from build123d import *

# Parameters (mm, degrees)
BOX_EXTRUDE_DEPTH                = 12.5
SHELL1_T                         = -3
CUT_SWEEP_START                  = -12.5
CUT_SWEEP_DEPTH                  = 4.5
SKETCH2_W                        = 10
SKETCH2_H                        = 10
SQUARES_EXTRUDE_DEPTH            = 9.5
SKETCH11_W                       = 10
SKETCH11_H                       = 31
SKETCH11_W_2                     = 45
SKETCH11_H_2                     = 10
CUT_EXTRUDE2_DEPTH               = 214.65503369
SQUARES_M3_CLEARANCE_HOLES_D     = 2.5
SQUARES_M3_CLEARANCE_HOLES_DEPTH = 2
SQUARES_M3_CLEARANCE_HOLES_TIP   = 0.751075774
F_8_0MM_DOWEL_HOLE1_D            = 8
F_8_0MM_DOWEL_HOLE1_DEPTH        = 7.5
F_8_0MM_DOWEL_HOLE1_TIP          = 2.403442476
F_5_0MM_DOWEL_HOLE1_D            = 5
F_5_0MM_DOWEL_HOLE1_DEPTH        = 7.5
F_5_0MM_DOWEL_HOLE1_TIP          = 1.502151548
M3_CLEARANCE_HOLE3_D             = 3.4
M3_CLEARANCE_HOLE3_DEPTH         = 7.5
M3_CLEARANCE_HOLE3_TIP           = 1.021463052
M3_5X0_6_TAPPED_HOLE1_D          = 2.9
M3_5X0_6_TAPPED_HOLE2_D          = 2.9
M3_5X0_6_TAPPED_HOLE2_DEPTH      = 8.8
M3_5X0_6_TAPPED_HOLE2_TIP        = 0.871247898
SKETCH25_W                       = 3
SKETCH25_H                       = 31
BOSS_EXTRUDE1_DEPTH              = 38.75
F_2_5MM_DOWEL_HOLE1_D            = 2.5
F_2_5MM_DOWEL_HOLE1_DEPTH        = 10
F_2_5MM_DOWEL_HOLE1_TIP          = 0.751075774


# Read off the part's stored shape, not the designer's step: Cut-Sweep
with BuildPart() as part:
    # Sketch1 → Box-Extrude (new body)
    with BuildSketch(Plane.XY):
        with BuildLine():
            Line((-64.633571826, -98.481365252), (179.366428174, -98.481365252))
            ThreePointArc((179.366428174, -98.481365252), (186.437495986, -95.552433064), (189.366428174, -88.481365252))
            Line((189.366428174, -88.481365252), (189.366428174, -8.481365252))
            ThreePointArc((189.366428174, -8.481365252), (186.437495986, -1.41029744), (179.366428174, 1.518634748))
            Line((179.366428174, 1.518634748), (-64.633571826, 1.518634748))
            ThreePointArc((-64.633571826, 1.518634748), (-71.704639638, -1.41029744), (-74.633571826, -8.481365252))
            Line((-74.633571826, -8.481365252), (-74.633571826, -88.481365252))
            ThreePointArc((-74.633571826, -88.481365252), (-71.704639638, -95.552433064), (-64.633571826, -98.481365252))
        make_face()
    extrude(amount=-BOX_EXTRUDE_DEPTH)

    # Shell1
    shell1_openings = [part.faces().sort_by_distance(p)[0] for p in [
        (57.366428174, -48.481365252, -12.5),
    ]]
    offset(amount=SHELL1_T, openings=shell1_openings, kind=Kind.INTERSECTION)

    # Cut-Sweep outline → Cut-Sweep (cut)
    with BuildSketch(Plane.XY.offset(CUT_SWEEP_START)):
        with BuildLine():
            Line((189.366428174, -88.481365252), (189.366428174, -8.481365252))
            ThreePointArc((189.366428174, -8.481365252), (186.437495986, -1.41029744), (179.366428174, 1.518634748))
            Line((179.366428174, 1.518634748), (-64.633571826, 1.518634748))
            ThreePointArc((-64.633571826, 1.518634748), (-71.704639638, -1.41029744), (-74.633571826, -8.481365252))
            Line((-74.633571826, -8.481365252), (-74.633571826, -88.481365252))
            ThreePointArc((-74.633571826, -88.481365252), (-71.704639638, -95.552433064), (-64.633571826, -98.481365252))
            Line((-64.633571826, -98.481365252), (179.366428174, -98.481365252))
            ThreePointArc((179.366428174, -98.481365252), (186.437495986, -95.552433064), (189.366428174, -88.481365252))
        make_face()
        with BuildLine():
            Line((179.366428174, -96.981365252), (-64.633571826, -96.981365252))
            ThreePointArc((-64.633571826, -96.981365252), (-70.643979466, -94.491772892), (-73.133571826, -88.481365252))
            Line((-73.133571826, -88.481365252), (-73.133571826, -8.481365252))
            ThreePointArc((-73.133571826, -8.481365252), (-70.643979466, -2.470957612), (-64.633571826, 0.018634748))
            Line((-64.633571826, 0.018634748), (179.366428174, 0.018634748))
            ThreePointArc((179.366428174, 0.018634748), (185.376835814, -2.470957612), (187.866428174, -8.481365252))
            Line((187.866428174, -8.481365252), (187.866428174, -88.481365252))
            ThreePointArc((187.866428174, -88.481365252), (185.376835814, -94.491772892), (179.366428174, -96.981365252))
        make_face(mode=Mode.SUBTRACT)
    extrude(amount=CUT_SWEEP_DEPTH, mode=Mode.SUBTRACT)

    # Sketch2 → Squares-Extrude (add)
    with BuildSketch(Plane.XY.offset(-3)):
        with Locations((41.816428174, -6.481365252)):
            Rectangle(SKETCH2_W, SKETCH2_H)
        with Locations((181.366428174, -65.481365252)):
            Rectangle(SKETCH2_W, SKETCH2_H)
        with Locations((41.366428174, -90.481365252)):
            Rectangle(SKETCH2_W, SKETCH2_H)
        with Locations((181.366428174, -31.481365252)):
            Rectangle(SKETCH2_W, SKETCH2_H)
    extrude(amount=-SQUARES_EXTRUDE_DEPTH)

    # Sketch11 → Cut-Extrude2 (cut, through all)
    with BuildSketch(Plane(origin=(0, 0, -3), x_dir=(-1, 0, 0), z_dir=(0, 0, -1))):
        with BuildLine():
            Line((-166.366428174, -66.481365252), (-110.366428174, -66.481365252))
            ThreePointArc((-110.366428174, -66.481365252), (-108.952214612, -65.895578814), (-108.366428174, -64.481365252))
            Line((-108.366428174, -64.481365252), (-108.366428174, -28.481365252))
            ThreePointArc((-108.366428174, -28.481365252), (-108.952214612, -27.067151689), (-110.366428174, -26.481365252))
            Line((-110.366428174, -26.481365252), (-166.366428174, -26.481365252))
            ThreePointArc((-166.366428174, -26.481365252), (-167.780641736, -27.067151689), (-168.366428174, -28.481365252))
            Line((-168.366428174, -28.481365252), (-168.366428174, -64.481365252))
            ThreePointArc((-168.366428174, -64.481365252), (-167.780641736, -65.895578814), (-166.366428174, -66.481365252))
        make_face()
        with Locations((62.633571826, -44.311365252)):
            Rectangle(SKETCH11_W, SKETCH11_H)
        with Locations((-152.769428174, 113.518634748)):
            Rectangle(SKETCH11_W_2, SKETCH11_H_2)
    extrude(amount=-CUT_EXTRUDE2_DEPTH, mode=Mode.SUBTRACT)

    # Squares M3 Clearance Holes
    with Locations(Plane(origin=(0, 0, -12.5), x_dir=(1, 0, 0), z_dir=(0, 0, -1))):
        with Locations((41.816428174, 6.481365252), (181.366428174, 31.481365252), (181.366428174, 65.481365252), (41.366428174, 90.481365252)):
            Hole(SQUARES_M3_CLEARANCE_HOLES_D / 2, depth=SQUARES_M3_CLEARANCE_HOLES_DEPTH)
            with Locations((0, 0, -(SQUARES_M3_CLEARANCE_HOLES_DEPTH + SQUARES_M3_CLEARANCE_HOLES_TIP / 2))):  # 118° drill point
                Cone(0, SQUARES_M3_CLEARANCE_HOLES_D / 2, SQUARES_M3_CLEARANCE_HOLES_TIP, mode=Mode.SUBTRACT)

    # Ø8.0mm Dowel Hole1
    with Locations(Plane(origin=(169.366428174, -85.481365252, -3), x_dir=(-1, 0, 0), z_dir=(0, 0, -1))):
        with Locations((0, 0), (31, 0), (62, 0), (71, 67), (-9, 67)):
            Hole(F_8_0MM_DOWEL_HOLE1_D / 2, depth=F_8_0MM_DOWEL_HOLE1_DEPTH)
            with Locations((0, 0, -(F_8_0MM_DOWEL_HOLE1_DEPTH + F_8_0MM_DOWEL_HOLE1_TIP / 2))):  # 118° drill point
                Cone(0, F_8_0MM_DOWEL_HOLE1_D / 2, F_8_0MM_DOWEL_HOLE1_TIP, mode=Mode.SUBTRACT)

    # Ø5.0mm Dowel Hole1
    with Locations(Plane(origin=(0, 0, -3), x_dir=(-1, 0, 0), z_dir=(0, 0, -1))):
        with Locations((-138.366428174, -22.481365252)):
            Hole(F_5_0MM_DOWEL_HOLE1_D / 2, depth=F_5_0MM_DOWEL_HOLE1_DEPTH)
            with Locations((0, 0, -(F_5_0MM_DOWEL_HOLE1_DEPTH + F_5_0MM_DOWEL_HOLE1_TIP / 2))):  # 118° drill point
                Cone(0, F_5_0MM_DOWEL_HOLE1_D / 2, F_5_0MM_DOWEL_HOLE1_TIP, mode=Mode.SUBTRACT)

    # M3 Clearance Hole3
    with Locations(Plane(origin=(0, 0, -3), x_dir=(-1, 0, 0), z_dir=(0, 0, -1))):
        with Locations((-163.366428174, -15.481365252), (-113.366428174, -15.481365252), (-163.366428174, -92.481365252), (-113.366428174, -92.481365252)):
            Hole(M3_CLEARANCE_HOLE3_D / 2, depth=M3_CLEARANCE_HOLE3_DEPTH)
            with Locations((0, 0, -(M3_CLEARANCE_HOLE3_DEPTH + M3_CLEARANCE_HOLE3_TIP / 2))):  # 118° drill point
                Cone(0, M3_CLEARANCE_HOLE3_D / 2, M3_CLEARANCE_HOLE3_TIP, mode=Mode.SUBTRACT)

    # M3.5x0.6 Tapped Hole1 (through all)
    with Locations(Plane(origin=(0, 0, -3), x_dir=(-1, 0, 0), z_dir=(0, 0, -1))):
        with Locations((-172.205915164, -24.061365252), (-172.205915164, -66.561365252), (-89.226428174, -25.561365252), (-89.226428174, -65.061365252), (-171.219428174, -11.481365252), (-131.719428174, -11.481365252)):
            Hole(M3_5X0_6_TAPPED_HOLE1_D / 2)

    # M3.5x0.6 Tapped Hole2
    with Locations(Plane.XY):
        with Locations((-66.633571826, -8.481365252), (-66.633571826, -88.481365252)):
            Hole(M3_5X0_6_TAPPED_HOLE2_D / 2, depth=M3_5X0_6_TAPPED_HOLE2_DEPTH)
            with Locations((0, 0, -(M3_5X0_6_TAPPED_HOLE2_DEPTH + M3_5X0_6_TAPPED_HOLE2_TIP / 2))):  # 118° drill point
                Cone(0, M3_5X0_6_TAPPED_HOLE2_D / 2, M3_5X0_6_TAPPED_HOLE2_TIP, mode=Mode.SUBTRACT)

    # Sketch25 → Boss-Extrude1 (add)
    with BuildSketch(Plane(origin=(0, 0, -3), x_dir=(-1, 0, 0), z_dir=(0, 0, -1))):
        with Locations((56.133571826, -44.311365252)):
            Rectangle(SKETCH25_W, SKETCH25_H)
    extrude(amount=BOSS_EXTRUDE1_DEPTH)

    # Ø2.5mm Dowel Hole1
    with Locations(Plane(origin=(-54.633571826, 0, 0), x_dir=(0, 0, -1), z_dir=(1, 0, 0))):
        with Locations((37.25, -32.811365252), (37.25, -55.811365252), (14.25, -32.811365252), (14.25, -55.811365252)):
            Hole(F_2_5MM_DOWEL_HOLE1_D / 2, depth=F_2_5MM_DOWEL_HOLE1_DEPTH)
            with Locations((0, 0, -(F_2_5MM_DOWEL_HOLE1_DEPTH + F_2_5MM_DOWEL_HOLE1_TIP / 2))):  # 118° drill point
                Cone(0, F_2_5MM_DOWEL_HOLE1_D / 2, F_2_5MM_DOWEL_HOLE1_TIP, mode=Mode.SUBTRACT)


solid = part.part
For this review, take the finished solid that the model builds, in its own axes (mm). A direction names the side the tool comes from. Give positions to 0.01 mm unless a question says otherwise; leave off trailing zeros. Loops run counter-clockwise (first coordinate to the right, second up) from the corner with the lowest first, then second, coordinate; pieces in that order, holes last. Notation, with made-up numbers: M -32,30 L -13,30 A25 cw -13,52 Z; hole C 87,41.25 d2. An arc over 180 degrees is marked long. Answer as a JSON object with one key per item and string values. Group by question number.
Q1. For probe 1 along X at (y, z) = (-47, -4.5); probe 2 along X at (y, z) = (-40.5, -10); probe 3 along Y at (x, z) = (-55, -14), list the stretches that pass through material, from the lowest coordinate up. Write a range as [from, to].
Q2. Add section C-C on z = -29. Give the boundary of the cut face in (x, y), and give its area (3 significant figures).
Q3. Tool access review of faces 1 (the flat face through (181, -36.481, -8)), 2 (the flat face through (-57.634, -45, -21)), 3 (the cylindrical face through (-70.71, -2.54, -10.28)), 4 (the flat face through (56, 0.019, -10)): name each direction out of +Z, -Z, +X, -X, +Y, -Y from which nothing blocks a thin tool from reaching the whole face with its end or side.
Q4. Insertion check: P1, Ø5, axis at x = 182.5, z = -6, coming from the +Y side; P2, Ø8, axis at x = 29.5, z = -16, coming from the +Y side; P3, Ø3, axis at y = -6, z = -8.5, coming from the +X side; P4, Ø6, axis at y = -25, z = -21.5, coming from the +X side. Each pin has a flat end and moves straight along its axis. Give the tip position at first contact, or say it passes through.
Q5. Add section B-B on x = 70.5. Give the boundary of the cut face in (y, z).
Q6. Mouldability with a two-part tool opening along X and no side actions: class faces 5 (the flat face through (59, 1.519, -4)), 6 (the flat face through (176.366, -32, -8)), 7 (the flat face through (187.866, -48, -10)), 8 (the flat face through (-73.134, -49, -10)) as +X half, -X half, draft (parallel to the pull), parting line (faces both ways), or undercut.
Q7. Add section A-A on y = -49.5. Give the boundary of the cut face in (x, z).
Checked values:
{
 "1": {"probe 1": "[-74.63, -71.63], [-57.63, -54.63], [186.37, 189.37]", "probe 2": "[-73.13, -71.63], [-57.63, -54.63], [186.37, 187.87]", "probe 3": "[-59.81, -57.04], [-54.59, -34.04], [-31.59, -28.81]"},
 "2": {"outline": "M -57.63,-59.81 L -54.63,-59.81 L -54.63,-28.81 L -57.63,-28.81 Z", "area": "93.0 mm²"},
 "3": {"face 1": "-Z", "face 2": "+Z, -Z", "face 3": "-Z, -X, +Y", "face 4": "-Z, +X, -X, +Y"},
 "4": {"P1": "y = 1.5", "P2": "y = 0.02", "P3": "x = 189.31", "P4": "through"},
 "5": {"outline": "M -98.48,-8 L -96.98,-8 L -96.98,-12.5 L -95.48,-12.5 L -95.48,-3 L -1.48,-3 L -1.48,-12.5 L 0.02,-12.5 L 0.02,-8 L 1.52,-8 L 1.52,0 L -98.48,0 Z"},
 "6": {"face 5": "draft", "face 6": "undercut", "face 7": "+X half", "face 8": "-X half"},
 "7": {"outline": "M -74.63,-8 L -73.13,-8 L -73.13,-12.5 L -71.63,-12.5 L -71.63,-3 L -67.63,-3 L -67.63,0 L -74.63,0 Z; M -57.63,-41.75 L -54.63,-41.75 L -54.63,-3 L 108.37,-3 L 108.37,0 L -57.63,0 Z; M 168.37,-3 L 186.37,-3 L 186.37,-12.5 L 187.87,-12.5 L 187.87,-8 L 189.37,-8 L 189.37,0 L 168.37,0 Z"}
}
